Autodesk Inventor part; units mm, degrees
ref_plane "WorkPlane1" through (0, 0, 0) normal (0, 0, 1) x (1, 0, 0)
ref_plane "Work Plane2" through (0, 0, -1) normal (0, 0, 1) x (1, 0, 0)
ref_plane "WorkPlane2" through (0, 0, 1.5) normal (0, 0, 1) x (1, 0, 0)
ref_plane "WorkPlane1" through (0, 0, 0) normal (0, 0, 1) x (1, 0, 0)
ref_plane "Work Plane2" through (0, 0, -1) normal (0, 0, 1) x (1, 0, 0)
ref_plane "WorkPlane2" through (0, 0, 1.5) normal (0, 0, 1) x (1, 0, 0)
sketch "Sketch1" plane through (0, 0, 0) normal (0, 0, 1) x (1, 0, 0)
  point P0 (0, 0)
sketch "Sketch2" plane through (0, 0, 0) normal (0, 0, 1) x (1, 0, 0)
  line L0 (4.25, -8.3873) -> (4.25, -5.4618)
  line L1 (0.85, -8.9868) -> (4.25, -8.3873)
  line L2 (0.85, -5.6868) -> (0.85, -8.9868)
  arc A0 (0.85, -5.6868) -> (-0.85, -5.6868) centre (0, 0) ccw
  line L3 (-0.85, -5.6868) -> (-0.85, -8.9868)
  line L4 (-0.85, -8.9868) -> (-4.25, -8.3873)
  line L5 (-4.25, -8.3873) -> (-4.25, -5.4618)
  arc A1 (4.25, -5.4618) -> (-4.25, -5.4618) centre (0, 0.35) ccw
  dimension "d2" = 5.75
  dimension "d4" = 7.2
  dimension "d6" = 0
  dimension "d8" = 0.85
  dimension "d10" = 0.85
  dimension "d12" = 3.3
  dimension "d14" = 3.3
  dimension "d16" = 80
  dimension "d18" = 80
  dimension "d20" = 3.4
  dimension "d22" = 3.4
  dimension "d24" = 0.35
  dimension "d52" = 0
  dimension "d53" = 0
extrude "Extrusion1" add sketch "Sketch2" along normal blind 1
sketch "Sketch3" plane through (0, 0, 1) normal (0, 0, 1) x (1, 0, 0)
  line L0 (-0.85, -5.6868) -> (-0.85, -8.9868)
  line L1 (-0.85, -8.9868) -> (-4.25, -8.3873)
  point P0 (-2.21, -7.2391)
  dimension "d30" = 1.36
  dimension "d32" = 1.485
hole "Hole1" at (-2.21, -7.2391, 1) direction (0, 0, -1) diameter 1.7 end through all
sketch "Sketch4" plane through (0, 0, 1) normal (0, 0, 1) x (1, 0, 0)
  line L0 (0.85, -8.9868) -> (0.85, -5.6868)
  line L1 (4.25, -8.3873) -> (0.85, -8.9868)
  point P0 (2.21, -7.2391)
  dimension "d41" = 1.36
  dimension "d43" = 1.485
hole "Hole2" at (2.21, -7.2391, 1) direction (0, 0, -1) diameter 1.7 end through all
fillet "Fillet1" radius 2.55 2 edges at (-4.25, -8.3873, 0.5) (4.25, -8.3873, 0.5)
equation "\"d33\" = Diam5"
equation "\"d44\" = Diam5"
equation "\"d51\" = 1.5 * Diam5"
equation "\"d2\" = 0.5 * Diam2"
equation "\"d4\" = 0.166667 * ParA + 0.5 * Diam2 + 0.5 * b"
equation "\"d8\" = 0.5 * Diam5"
equation "\"d10\" = 0.5 * Diam5"
equation "\"d12\" = ParA"
equation "\"d14\" = ParA"
equation "\"d20\" = 2 * Diam5"
equation "\"d22\" = 2 * Diam5"
equation "\"d24\" = -msp_r2 + 0.5 * Diam2 + b"
equation "\"d25\" = ParS"
equation "\"Diam5\" = 1.7"
equation "\"ParA\" = 3.3"
equation "\"ParS\" = 1"
equation "\"Diam2\" = 11.5"
equation "\"msp_r2\" = 0.166667 * ParA + 0.5 * Diam2 + 0.5 * b"
equation "\"TEMPLATE\" = 1.2345"
properties part number "DIN 471 - 12x1" material "Steel, Mild"
Read the model definition and answer for the solid it produces. Units are mm, in the model's axes. A direction names the side the tool comes from. Give positions to 0.01 mm unless a question says otherwise; leave off trailing zeros. Write each loop counter-clockwise with the first axis right and the second up, starting at its lowest first coordinate (ties: lowest second). Pieces come first, ordered by that corner, then holes. Notation, with made-up numbers: (-20.75, -9.75) -> (18.25, -9.75) arc R14 cw to (18.25, 5.25) -> close; hole circle Ø10 at (-0.5, 43.5). An arc over 180 degrees is marked (long way). Answer in a Markdown table with one row per item.
1) Determine the mould class of faces 1 (the cylindrical face through (-0.241, 5.745, 0.493)), 2 (the flat face through (-1.487, -8.874, 0.493)), 3 (the flat face through (0.85, -7.3, 0.5)) for opening direction Y: released by +Y, released by -Y, zero draft, split by the parting line, or undercut.
Results list:
| item | result |
|---|---|
| face 1 | undercut |
| face 2 | released by -Y |
| face 3 | zero draft |
2) Section B-B on x = -4.5 is taken. Give the vertices of the cut face in (y, z), plus the area to 3 significant figures.
Results list:
| item | result |
|---|---|
| outline | (-5.27, 0) -> (-3.58, 0) -> (-3.58, 1) -> (-5.27, 1) -> close; (3.58, 0) -> (5.97, 0) -> (5.97, 1) -> (3.58, 1) -> close |
| area | 4.08 mm^2 |
3) Each of these flat-tipped pins is pushed along its axis until it touches: pin 1 Ø1.5 at (x, y) = (2.21, -7.24) entering from -Z; pin 2 Ø3 at (x, y) = (5, -2) entering from -Z; pin 3 Ø0.5 at (y, z) = (-7, 0.5) entering from -X; pin 4 Ø0.6 at (y, z) = (-6, 0.5) entering from +X. Where does it stop, or does it pass through?
Results list:
| item | result |
|---|---|
| pin 1 | through |
| pin 2 | z = 0 |
| pin 3 | x = -4.2 |
| pin 4 | x = 4.25 |
4) A tool of negligible diameter and unlimited length cuts with its end or side. For faces 4 (the flat face through (-0.85, -7.3, 0.5)), 5 (the cylindrical face through (-3.669, -7.868, 0.507)), from which of +Z, -Z, +X, -X, +Y, -Y can it reach the whole face along a straight path? Write none if from no direction.
Results list:
| item | result |
|---|---|
| face 4 | +Z, -Z, -Y |
| face 5 | +Z, -Z, -X, -Y |
5) Section D-D on y = -2.25 is taken. Give the vertices of the cut face in (x, z).
Results list:
| item | result |
|---|---|
| outline | (-6.71, 0) -> (-5.29, 0) -> (-5.29, 1) -> (-6.71, 1) -> close; (5.29, 0) -> (6.71, 0) -> (6.71, 1) -> (5.29, 1) -> close |
6) Section A-A on z = 0.4 is taken. Give the vertices of the cut face in (x, y).
Results list:
| item | result |
|---|---|
| outline | (-4.25, -6.25) arc R2.55 ccw to (-2.14, -8.76) -> (-0.85, -8.99) -> (-0.85, -5.69) arc R5.75 cw (long way) to (0.85, -5.69) -> (0.85, -8.99) -> (2.14, -8.76) arc R2.55 ccw to (4.25, -6.25) -> (4.25, -5.46) arc R7.2 ccw (long way) to (-4.25, -5.46) -> close; hole circle Ø1.7 at (-2.21, -7.24); hole circle Ø1.7 at (2.21, -7.24) |
7) Straight lines are drawn through the part: line 1 (Y direction, x = -2.21, z = 0.2); line 2 (X direction, y = -7.5, z = 0.5); line 3 (X direction, y = -6.25, z = 0.75). For each, find the intervals that lie inside material, in ascending order. Write a range as [from, to].
Results list:
| item | result |
|---|---|
| line 1 | [-8.75, -8.09], [-6.39, -5.31], [5.31, 7.2] |
| line 2 | [-3.92, -3.02], [-1.4, -0.85], [0.85, 1.4], [3.02, 3.92] |
| line 3 | [-4.25, -0.85], [0.85, 4.25] |
8) Section C-C on y = -6.75 is taken. Give the vertices of the cut face in (x, z).
Results list:
| item | result |
|---|---|
| outline | (-4.2, 0) -> (-2.91, 0) -> (-2.91, 1) -> (-4.2, 1) -> close; (-1.51, 0) -> (-0.85, 0) -> (-0.85, 1) -> (-1.51, 1) -> close; (0.85, 0) -> (1.51, 0) -> (1.51, 1) -> (0.85, 1) -> close; (2.91, 0) -> (4.2, 0) -> (4.2, 1) -> (2.91, 1) -> close |
